Answer from the drawing. Dimensions are ordinates in mm from the lowest x, y and z of the part. Give positions to 0.01 mm unless a question says otherwise; leave off trailing zeros. Order: outer loops, then holes, each group sorted by start corner. A loop starts at its lowest first (then second) coordinate and runs counter-clockwise, first axis right, second up. Notation, with made-up numbers: (16, -16) - (22, -16) arc R23 cw to (22, 13) - close; hole circle Ø9 at (73.25, 17.5). An arc over 180 degrees is marked (long way). Use a Markdown table: item, result. Add a question column.
1) Flat-ended cylindrical pins translate along their axes: pin 1 (10.5 mm diameter, centred on y = 12.5, z = 69.5, fed in from -X); pin 2 (10.5 mm diameter, centred on y = 25, z = 56, fed in from +X). Find the tip coordinate at first contact, or state that the pin passes through.
2) A straight line is drawn through the part: line 1 (X direction, y = 30, z = 77.5). Find the intervals that lie inside material, in ascending order.
3) Find section B-B, the plane z = 40.5. Determine the outline of the cut face in (x, y).
4) Find section A-A, the plane y = 30. Determine the outline of the cut face in (x, z).
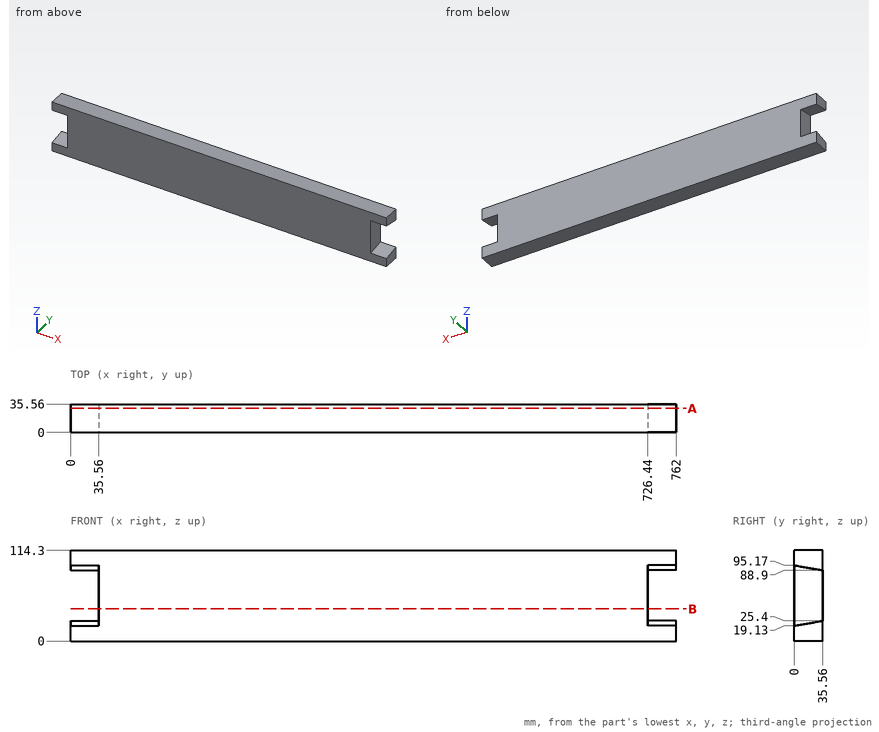
The answers:
| question | item | result |
|---|---|---|
| 1 | pin 1 | x = 35.56 |
| 1 | pin 2 | x = 726.44 |
| 2 | line 1 | 35.56 to 726.44 |
| 3 | outline | (35.56, 0) - (726.44, 0) - (726.44, 35.56) - (35.56, 35.56) - close |
| 4 | outline | (0, 0) - (762, 0) - (762, 24.42) - (726.44, 24.42) - (726.44, 89.88) - (762, 89.88) - (762, 114.3) - (0, 114.3) - (0, 89.88) - (35.56, 89.88) - (35.56, 24.42) - (0, 24.42) - close |
